Input: part model. Units: mm. Frame: model coordinates. A direction names the side the tool comes from. Round coordinates to 2 decimals unless told otherwise and drop trailing zeros. Loops run counter-clockwise (first coordinate to the right, second up) from the corner with the lowest first, then second, coordinate; pieces in that order, holes last. Notation, with made-up numbers: M 13,40.5 L 57,40.5 A19 cw 57,68.5 Z; hole C -29.5,45.5 d5. An arc over 180 degrees is marked long. Return JSON: item names as keys, results as strings. Group by question number.
1) Section C-C (z = -4.5). Output: boundary loops of the cut face in (x, y).
2) Contact query for flat-ended pins moving along their axis: P1, Ø1.5, axis at x = 2, z = 7, coming from the -Y side; P2, Ø2, axis at x = 5.66, y = -5.66, coming from the +Z side; P3, Ø6, axis at y = 13, z = -1, coming from the +X side. Output: stop coordinate, or through.
3) Section D-D (z = 14.5). Output: boundary loops of the cut face in (x, y).
4) Section B-B (y = 0). Output: boundary loops of the cut face in (x, z).
5) Material intervals for line 1 (Z direction, x = 18, y = -16.5); line 2 (X direction, y = 4.5, z = -6.5); line 3 (Z direction, x = 16.5, y = 10.5), sorted ascending. Write a range as from..to.
6) Mould query, pull axis X, two halves, no side actions, for faces 6 (the face through (-11, 4, -16)), 7 (the face through (-20.68, 15.094, 0.224)), 8 (the face through (-6, 12, -8)), 9 (the face through (22.961, -11, 0)). Classes: +X half, -X half, draft (parallel to the pull), parting line (faces both ways), or undercut.
7) Access query for faces 1 (the face through (17.761, 0, 8)), 2 (the face through (-12, -14, 10)), 3 (the face through (-22.961, -11, 0)), 4 (the face through (-5.73, 3.96, -10.03)), 5 (the face through (6.067, 14, 0)). Directions: +Z, -Z, +X, -X, +Y, -Y. A direction counts if a zero-diameter tool reaches every point of the face in a straight line with its end or side. Return the directions, or none.
8) Section A-A (x = 0). Output: boundary loops of the cut face in (y, z).
from build123d import *

# Parameters (mm, degrees)
SKETCH1_W                = 45.922011884
SKETCH1_H                = 35
BOSS_EXTRUDE1_DEPTH      = 16
CUT_EXTRUDE1_DEPTH       = 34.006935542
CUT_EXTRUDE1_DEPTH_BACK  = 34.006935542
SKETCH2_R                = 4.1
CUT_EXTRUDE2_REACH       = 45.098
SKETCH4_W                = 5
SKETCH4_H                = 10
CUT_EXTRUDE3_DEPTH       = 10
SKETCH6_R                = 11.2
CUT_EXTRUDE4_DEPTH       = 4
SKETCH7_R                = 5.1
CUT_EXTRUDE5_DEPTH       = 10.5
CIRPATTERN1_COUNT        = 2
CUT_EXTRUDE6_DEPTH       = 34.006935542
CUT_EXTRUDE6_DEPTH_BACK  = 34.006935542
SKETCH8_R                = 3.2
FILLET1_R                = 8
CUT_EXTRUDE8_START       = -4
SKETCH9_R                = 5.1
CUT_EXTRUDE8_DEPTH       = 2.6
CIRPATTERN2_COUNT        = 2
SKETCH13_W               = 32.238994058
SKETCH13_H               = 10.4
CUT_REVOLVE1_ANGLE       = 90
SKETCH14_R               = 10
CUT_EXTRUDE9_DEPTH       = 5.5
CUT_EXTRUDE10_DEPTH      = 44.098234306
CUT_EXTRUDE11_START      = -3
CUT_EXTRUDE11_DEPTH      = 2.6
M3_CLEARANCE_HOLE2_D     = 3.4
M3_CLEARANCE_HOLE2_DEPTH = 10
M3_CLEARANCE_HOLE2_TIP   = 1.021463052


with BuildPart() as part:
    # Sketch1 → Boss-Extrude1 (new, symmetric)
    with BuildSketch(Plane.XY):
        Rectangle(SKETCH1_W, SKETCH1_H)
    extrude(amount=BOSS_EXTRUDE1_DEPTH, both=True)

    # Sketch2 → Cut-Extrude1 (cut, two sides: drawn at the far end of the back side and taken through both)
    with BuildSketch(Plane.XY.offset(-CUT_EXTRUDE1_DEPTH_BACK)):
        Circle(SKETCH2_R)
    extrude(amount=CUT_EXTRUDE1_DEPTH + CUT_EXTRUDE1_DEPTH_BACK, mode=Mode.SUBTRACT)

    # Sketch4 → Cut-Extrude2 (cut, up to next)
    with BuildSketch(Plane.XY.offset(16), mode=Mode.PRIVATE) as cut_extrude2_sk1:
        with Locations((20.461005942, 0)):
            Rectangle(SKETCH4_W, SKETCH4_H)
    cut_extrude2_tool1 = extrude(cut_extrude2_sk1.sketch, amount=-CUT_EXTRUDE2_REACH, mode=Mode.PRIVATE) & part.part
    # Sketch4 → Cut-Extrude2 (cut, up to next)
    with BuildSketch(Plane.XY.offset(16), mode=Mode.PRIVATE) as cut_extrude2_sk2:
        with Locations((-20.461005942, 0)):
            Rectangle(SKETCH4_W, SKETCH4_H)
    cut_extrude2_tool2 = extrude(cut_extrude2_sk2.sketch, amount=-CUT_EXTRUDE2_REACH, mode=Mode.PRIVATE) & part.part
    # Sketch4 → Cut-Extrude2 (cut, up to next)
    with BuildSketch(Plane.XY.offset(16), mode=Mode.PRIVATE) as cut_extrude2_sk3:
        Polygon((17.961005942, 5), (22.961005942, 5), (22.961005942, 5.2), (17.761005942, 5.2), (17.761005942, -5.2), (22.961005942, -5.2), (22.961005942, -5), (17.961005942, -5), align=None)
    cut_extrude2_tool3 = extrude(cut_extrude2_sk3.sketch, amount=-CUT_EXTRUDE2_REACH, mode=Mode.PRIVATE) & part.part
    # Sketch4 → Cut-Extrude2 (cut, up to next)
    with BuildSketch(Plane.XY.offset(16), mode=Mode.PRIVATE) as cut_extrude2_sk4:
        Polygon((-22.961005942, 5.2), (-22.961005942, 5), (-17.961005942, 5), (-17.961005942, -5), (-22.961005942, -5), (-22.961005942, -5.2), (-17.761005942, -5.2), (-17.761005942, 5.2), align=None)
    cut_extrude2_tool4 = extrude(cut_extrude2_sk4.sketch, amount=-CUT_EXTRUDE2_REACH, mode=Mode.PRIVATE) & part.part
    add(cut_extrude2_tool1.solids().sort_by_distance((20.461006, 0, 16))[0], mode=Mode.SUBTRACT)
    add(cut_extrude2_tool2.solids().sort_by_distance((-20.461006, 0, 16))[0], mode=Mode.SUBTRACT)
    add(cut_extrude2_tool3.solids().sort_by_distance((17.84473, 0, 16))[0], mode=Mode.SUBTRACT)
    add(cut_extrude2_tool4.solids().sort_by_distance((-22.84473, 5.1, 16))[0], mode=Mode.SUBTRACT)

    # Sketch5 → Cut-Extrude3 (cut, symmetric)
    # profile 1 of 2: a face of its own
    with BuildSketch(Plane.XY):
        with BuildLine():
            Line((6.067449647, 17.6), (6.067449647, 9.762846361))
            ThreePointArc((6.067449647, 9.762846361), (12.167449647, 3.662846361), (18.267449647, 9.762846361))
            Line((18.267449647, 9.762846361), (18.267449647, 17.6))
            Line((18.267449647, 17.6), (6.067449647, 17.6))
        make_face()
        with BuildLine():
            ThreePointArc((6.167449647, 9.762846361), (12.167449647, 3.762846361), (18.167449647, 9.762846361))
            Line((18.167449647, 9.762846361), (18.167449647, 17.5))
            Line((18.167449647, 17.5), (6.167449647, 17.5))
            Line((6.167449647, 17.5), (6.167449647, 9.762846361))
        make_face(mode=Mode.SUBTRACT)
    # profile 2 of 2: a face of its own
    with BuildSketch(Plane.XY):
        with BuildLine():
            Line((6.167449647, 17.5), (6.167449647, 9.762846361))
            ThreePointArc((6.167449647, 9.762846361), (12.167449647, 3.762846361), (18.167449647, 9.762846361))
            Line((18.167449647, 9.762846361), (18.167449647, 17.5))
            Line((18.167449647, 17.5), (6.167449647, 17.5))
        make_face()
    cut_extrude3 = extrude(amount=CUT_EXTRUDE3_DEPTH, both=True, mode=Mode.SUBTRACT)

    # Sketch6 → Cut-Extrude4 (cut)
    with BuildSketch(Plane(origin=(0, 0, -16), x_dir=(-1, 0, 0), z_dir=(0, 0, -1))):
        Circle(SKETCH6_R)
    extrude(amount=-CUT_EXTRUDE4_DEPTH, mode=Mode.SUBTRACT)

    # Sketch7 → Cut-Extrude5 (cut)
    with BuildSketch(Plane(origin=(0, 0, -12), x_dir=(-1, 0, 0), z_dir=(0, 0, -1))):
        Circle(SKETCH7_R)
    extrude(amount=-CUT_EXTRUDE5_DEPTH, mode=Mode.SUBTRACT)

    # CirPattern1: Cut-Extrude3 ×2 about axis
    cirpattern1_axis = Axis((0, 0, 0), (0, 0, 1))
    for i in range(1, CIRPATTERN1_COUNT):
        add(cut_extrude3.rotate(cirpattern1_axis, i * 360 / CIRPATTERN1_COUNT), mode=Mode.SUBTRACT)

    # Sketch8 → Cut-Extrude6 (cut, two sides: drawn at the far end of the back side and taken through both)
    with BuildSketch(Plane.XY.offset(-CUT_EXTRUDE6_DEPTH_BACK)):
        with Locations((-12.167449647, -9.762846361)):
            Circle(SKETCH8_R)
        with Locations((12.167449647, 9.762846361)):
            Circle(SKETCH8_R)
    extrude(amount=CUT_EXTRUDE6_DEPTH + CUT_EXTRUDE6_DEPTH_BACK, mode=Mode.SUBTRACT)

    # Fillet1
    # the kernel refuses this fillet: 8 mm, written as the material it takes off along each edge
    with BuildSketch(Plane(origin=(22.961005942, 17.5, -36), x_dir=(-1, 0, 0), z_dir=(0, 0, 1))) as fillet1_piece_1:
        with BuildLine():
            CenterArc((FILLET1_R, FILLET1_R), FILLET1_R, 180, 90)
            Line((0, FILLET1_R), (0, 0))
            Line((0, 0), (FILLET1_R, 0))
        make_face()
    extrude(amount=72, mode=Mode.SUBTRACT)
    with BuildSketch(Plane(origin=(-22.961005942, 17.5, 36), x_dir=(0, -1, 0), z_dir=(0, 0, -1))) as fillet1_piece_2:
        with BuildLine():
            CenterArc((FILLET1_R, -FILLET1_R), FILLET1_R, 90, 90)
            Line((0, -FILLET1_R), (0, 0))
            Line((0, 0), (FILLET1_R, 0))
        make_face()
    extrude(amount=72, mode=Mode.SUBTRACT)

    # Sketch9 → Cut-Extrude8 (cut)
    with BuildSketch(Plane(origin=(0, 0, -12), x_dir=(-1, 0, 0), z_dir=(0, 0, -1)).offset(CUT_EXTRUDE8_START)):
        with BuildLine():
            Line((2.856854249, 17.5), (2.856854249, 10.829514477))
            ThreePointArc((2.856854249, 10.829514477), (5.919350665, 9.507959177), (8.456854249, 7.34313395))
            Line((8.456854249, 7.34313395), (8.456854249, 17.5))
            Line((8.456854249, 17.5), (2.856854249, 17.5))
        make_face()
        Circle(SKETCH9_R)
        Polygon((2.856854249, 4.040273496), (5.656854249, 2.423692742), (8.456854249, 4.040273496), (8.456854249, 7.273435003), (5.656854249, 8.890015757), (2.856854249, 7.273435003), align=None)
        with BuildLine():
            Line((2.856854249, 10.829514477), (2.856854249, 7.273435003))
            Line((2.856854249, 7.273435003), (5.656854249, 8.890015757))
            Line((5.656854249, 8.890015757), (8.456854249, 7.273435003))
            Line((8.456854249, 7.273435003), (8.456854249, 7.34313395))
            ThreePointArc((8.456854249, 7.34313395), (5.919350665, 9.507959177), (2.856854249, 10.829514477))
        make_face()
    cut_extrude8 = extrude(amount=-CUT_EXTRUDE8_DEPTH, mode=Mode.SUBTRACT)

    # Sketch11 → M3 Clearance Hole1 (revolve, cut)
    with BuildSketch(Plane(origin=(-5.656854249, 5.656854249, -12), x_dir=(0, 1, 0), z_dir=(1, 0, 0))):
        Polygon((0, 0), (0, 11.021463052), (1.7, 10), (1.7, 0), align=None)
    m3_clearance_hole1 = revolve(axis=Axis((-5.656854249, 5.656854249, -18.35), (0, 0, 1)), mode=Mode.SUBTRACT)

    # CirPattern2: Cut-Extrude8, M3 Clearance Hole1 ×2 about axis
    cirpattern2_axis = Axis((0, 0, 0), (0, 0, 1))
    add([cut_extrude8.rotate(cirpattern2_axis, i * 360 / CIRPATTERN2_COUNT) for i in range(1, CIRPATTERN2_COUNT)], mode=Mode.SUBTRACT)
    add([m3_clearance_hole1.rotate(cirpattern2_axis, i * 360 / CIRPATTERN2_COUNT) for i in range(1, CIRPATTERN2_COUNT)], mode=Mode.SUBTRACT)

    # Sketch13 → Cut-Revolve1 (revolve, cut)
    with BuildSketch(Plane.XY):
        with Locations((33.880502971, 0)):
            Rectangle(SKETCH13_W, SKETCH13_H)
        with Locations((-33.880502971, 0)):
            Rectangle(SKETCH13_W, SKETCH13_H)
    revolve(axis=Axis((0, 0, 0), (0, 1, 0)), revolution_arc=CUT_REVOLVE1_ANGLE, mode=Mode.SUBTRACT)

    # Sketch14 → Cut-Extrude9 (cut)
    with BuildSketch(Plane.XY.offset(16)):
        Circle(SKETCH14_R)
    extrude(amount=-CUT_EXTRUDE9_DEPTH, mode=Mode.SUBTRACT)

    # Sketch15 → Cut-Extrude10 (cut, through all)
    with BuildSketch(Plane.XY.offset(16)):
        Polygon((-4, -17.5), (-5.5, -13.5), (5.5, -13.5), (4, -17.5), align=None)
    extrude(amount=-CUT_EXTRUDE10_DEPTH, mode=Mode.SUBTRACT)

    # Sketch16 → Cut-Extrude11 (cut)
    with BuildSketch(Plane.XZ.offset(17.5).offset(CUT_EXTRUDE11_START)):
        Polygon((19.616580754, -2.8), (21.233161507, 0), (19.616580754, 2.8), (16.383419246, 2.8), (14.766838493, 0), (16.383419246, -2.8), align=None)
        Polygon((21.233161507, 0), (19.616580754, -2.8), (22.961005942, -2.8), (22.961005942, 2.8), (19.616580754, 2.8), align=None)
    extrude(amount=-CUT_EXTRUDE11_DEPTH, mode=Mode.SUBTRACT)

    # M3 Clearance Hole2
    with Locations(Plane(origin=(0, -17.5, 0), x_dir=(-1, 0, 0), z_dir=(0, -1, 0))):
        with Locations((-18, 0)):
            Hole(M3_CLEARANCE_HOLE2_D / 2, depth=M3_CLEARANCE_HOLE2_DEPTH)
            with Locations((0, 0, -(M3_CLEARANCE_HOLE2_DEPTH + M3_CLEARANCE_HOLE2_TIP / 2))):  # 118° drill point
                Cone(0, M3_CLEARANCE_HOLE2_D / 2, M3_CLEARANCE_HOLE2_TIP, mode=Mode.SUBTRACT)


solid = part.part
Returned:
{
 "1": {"outline": "M -22.96,-17.5 L -18.27,-17.5 L -18.27,-9.76 A6.1 cw -6.07,-9.76 L -6.07,-17.5 L -4,-17.5 L -5.5,-13.5 L 5.5,-13.5 L 4,-17.5 L 22.96,-17.5 L 22.96,-5.2 L 17.18,-5.2 L 17.18,5.2 L 22.96,5.2 L 22.96,9.5 A8 ccw 18.27,16.78 L 18.27,9.76 A6.1 cw 6.07,9.76 L 6.07,17.5 L -14.96,17.5 A8 ccw -22.96,9.5 L -22.96,5.2 L -17.76,5.2 L -17.76,-5.2 L -22.96,-5.2 Z; hole C -5.66,5.66 d3.4; hole C 0,0 d10.2; hole C 5.66,-5.66 d3.4"},
 "2": {"P1": "stops at y = -13.5", "P2": "stops at z = 10.5", "P3": "stops at x = 22.95"},
 "3": {"outline": "M -22.96,-17.5 L -4,-17.5 L -5.5,-13.5 L 5.5,-13.5 L 4,-17.5 L 22.96,-17.5 L 22.96,-5.2 L 17.76,-5.2 L 17.76,5.2 L 22.96,5.2 L 22.96,9.5 A8 ccw 14.96,17.5 L -14.96,17.5 A8 ccw -22.96,9.5 L -22.96,5.2 L -10.26,5.2 L -10.26,-5.2 L -22.96,-5.2 Z; hole C -12.17,-9.76 d6.4; hole C 0,0 d20; hole C 12.17,9.76 d6.4"},
 "4": {"outline": "M -17.76,-16 L -11.2,-16 L -11.2,-12 L -5.1,-12 L -5.1,-1.5 L -4.1,-1.5 L -4.1,10.5 L -10,10.5 L -10,14.68 A17.76 ccw -17.76,0 Z; M 4.1,-1.5 L 5.1,-1.5 L 5.1,-12 L 11.2,-12 L 11.2,-13.78 A17.76 ccw 17.76,0 L 17.76,16 L 10,16 L 10,10.5 L 4.1,10.5 Z"},
 "5": {"line 1": "z = -16..-1.7, 1.7..16", "line 2": "x = -17.76..-8.46, -2.86..-2.4, 2.4..9.08, 15.25..16.53", "line 3": "z = -16..-10, 10..16"},
 "6": {"face 6": "draft", "face 7": "-X half", "face 8": "undercut", "face 9": "+X half"},
 "7": {"face 1": "+Z, -Z, +X", "face 2": "-Y", "face 3": "+Z, -Z, -X, +Y, -Y", "face 4": "-Z", "face 5": "+Y"},
 "8": {"outline": "M -13.5,-16 L -11.2,-16 L -11.2,-12 L -5.1,-12 L -5.1,-1.5 L -4.1,-1.5 L -4.1,10.5 L -10,10.5 L -10,16 L -13.5,16 Z; M 4.1,-1.5 L 5.1,-1.5 L 5.1,-12 L 11.2,-12 L 11.2,-16 L 17.5,-16 L 17.5,16 L 10,16 L 10,10.5 L 4.1,10.5 Z"}
}
